Read the model definition and answer for the solid it produces. Units are mm, in the model's axes. Face numbers are marked on the shaded views. A direction names the side the tool comes from. Give positions to 0.01 mm unless a question says otherwise; leave off trailing zeros. Order: outer loops, then holes, each group sorted by start corner. A loop starts at its lowest first (then second) coordinate and runs counter-clockwise, first axis right, second up.
Item 1: Given pin 1 Ø1.5 at (x, z) = (-63, -4) entering from +Y, flat-ended and moving along its own axis, determine where the tip first touches the part or whether it passes through.
Item 2: A cutting plane is placed at C-C (z = -13). Write down the section's boundary in (x, y) (1 decimal).
Item 3: Find the intervals of material crossed by line 1 along X through (y, z) = (-98, -17); line 2 along Z through (x, y) = (-74, -121); line 3 along X through (y, z) = (-75.5, -37), in increasing order.
Item 4: A cutting plane is placed at B-B (x = 20.5). Write down the section's boundary in (y, z) (3 decimals), plus the area to 3 significant figures.
Item 5: The mould has two halves that part along Z. Classify the marked faces 1, 2 and 3: +Z half, -Z half, draft (parallel to the pull), parting line (faces both ways), or undercut.
Item 6: A cutting plane is placed at A-A (y = -76.5). State how many separate pieces and enclosed holes the cut face has, plus the area to 3 significant figures.
Item 7: A cutting plane is placed at D-D (x = -75.5). Write down the section's boundary in (y, z) (3 decimals), plus the area to 3 significant figures.
Item 8: Which of the six approach directions +Z, -Z, +X, -X, +Y, -Y give full straight-line access (tool end or side, diameter ignored) to the marked faces 4 and 5?
from build123d import *

# Parameters (mm, degrees)
F0_W     = 149.225
F0_H     = 76.2
F0_W_2   = 47.625
F0_H_2   = 34.925
F0_W_3   = 31.75
F0_H_3   = 19.05
F0_H_4   = 25.4
F0_H_5   = 31.75
F0_W_4   = 50.8
F1_DEPTH = 127
F2_W     = 149.225
F2_H     = 76.2
F3_DEPTH = 3.175


# Not quite as in the source:
# - a length typed as a fraction of an inch, garbled in the dataset ("3 / 203.2 mm" for 3/8 in), is restored


with BuildPart() as f1:
    # F0 (on Front) → F1 (new body)
    with BuildSketch(Plane.XZ):
        with Locations((-19.0595093454, -28.2635252237)):
            Rectangle(F0_W, F0_H)
        with Locations((-68.2720093454, -45.7260252237)):
            Rectangle(F0_W_2, F0_H_2, mode=Mode.SUBTRACT)
        with Locations((-19.2011359204, -31.6498865128)):
            Rectangle(F0_W_3, F0_H_3, mode=Mode.SUBTRACT)
        with Locations((-19.0595093454, -53.6635252237)):
            Rectangle(F0_W_2, F0_H_3, mode=Mode.SUBTRACT)
        with Locations((30.1529906546, -50.4885252237)):
            Rectangle(F0_W_2, F0_H_4, mode=Mode.SUBTRACT)
        with Locations((-76.2095093454, -9.2135252237)):
            Rectangle(F0_W_3, F0_H_5, mode=Mode.SUBTRACT)
        with Locations((-25.4095093454, -6.0385252237)):
            Rectangle(F0_W_4, F0_H_4, mode=Mode.SUBTRACT)
        with Locations((28.5654906546, -6.0385252237)):
            Rectangle(F0_W_4, F0_H_4, mode=Mode.SUBTRACT)
    extrude(amount=F1_DEPTH)

    # F2 (on face) → F3 (join)
    with BuildSketch(Plane.XZ.offset(127)):
        with Locations((-19.0595093454, -28.2635252237)):
            Rectangle(F2_W, F2_H)
    extrude(amount=F3_DEPTH)


solid = f1.part
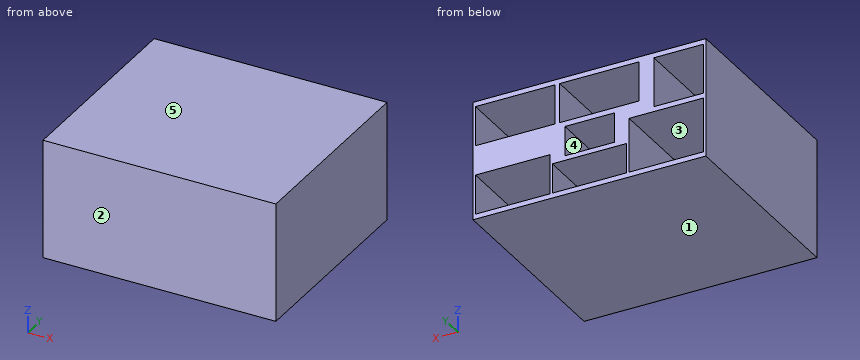
Response values:
1. pin 1: stops at y = -127
2. outline: (-93.7, -130.2) - (55.6, -130.2) - (55.6, 0) - (54, 0) - (54, -127) - (3.2, -127) - (3.2, 0) - (0, 0) - (0, -127) - (-50.8, -127) - (-50.8, 0) - (-60.3, 0) - (-60.3, -127) - (-92.1, -127) - (-92.1, 0) - (-93.7, 0) - close
3. line 1: x = -93.67 to -92.08, -60.33 to -50.81, -0.01 to 3.17, 53.97 to 55.55
3. line 2: z = -66.36 to -63.19, -28.26 to -25.09, 6.66 to 9.84
3. line 3: x = -93.67 to -92.08, -44.46 to -35.08, -3.33 to 55.55
4. outline: (-130.175, -66.364) - (0, -66.364) - (0, -63.189) - (-127, -63.189) - (-127, -37.789) - (0, -37.789) - (0, -18.739) - (-127, -18.739) - (-127, 6.661) - (0, 6.661) - (0, 9.836) - (-130.175, 9.836) - close
4. area: 3,470 mm2
5. face 1: -Z half
5. face 2: draft
5. face 3: undercut
6. separate pieces: 1
6. enclosed holes: 7
6. area: 3,400 mm2
7. outline: (-130.175, -66.364) - (0, -66.364) - (0, -63.189) - (-127, -63.189) - (-127, -28.264) - (0, -28.264) - (0, -25.089) - (-127, -25.089) - (-127, 6.661) - (0, 6.661) - (0, 9.836) - (-130.175, 9.836) - close
7. area: 1,450 mm2
8. face 4: +Y
8. face 5: +Z, +X, -X, +Y, -Y
